Design review of the part built by this model. Coordinates are the model's own, in mm. A direction names the side the tool comes from. Give positions to 0.01 mm unless a question says otherwise; leave off trailing zeros. Order: outer loops, then holes, each group sorted by start corner. A loop starts at its lowest first (then second) coordinate and runs counter-clockwise, first axis right, second up. Notation, with made-up numbers: (-33.5, 82) -> (8.5, 82) arc R30 cw to (8.5, 106) -> close; hole circle Ø10 at (27.5, 12.25). An arc over 180 degrees is marked (long way). One line per item, written item: value.
from build123d import *

# Parameters (mm, degrees)
SKETCH4_W              = 63.5
SKETCH4_H              = 54.9275
BASE_FLANGE1_DEPTH     = 1.905
SKETCHED_START         = -31.75
SKETCHED_BEND3_DEPTH   = 63.5
SKETCHED_BEND3_2_DEPTH = 63.5
CUT_EXTRUDE2_REACH     = 51.835
SKETCH20_R             = 2


# Read off the part's stored shape, not the designer's step: Sketched Bend3
# Sheet-metal steps are written as plain solids
with BuildPart() as part:
    # Sketch4 → Base-Flange1 (new body)
    with BuildSketch(Plane(origin=(0, 0, 0), x_dir=(0, 0, -1), z_dir=(1, 0, 0))):
        Rectangle(SKETCH4_W, SKETCH4_H)
    extrude(amount=-BASE_FLANGE1_DEPTH)

    # Sketched Bend3 outline → Sketched Bend3 (cut)
    with BuildSketch(Plane.XY.offset(SKETCHED_START)):
        with BuildLine():
            ThreePointArc((0, -18.310223013), (-1.375727285, -17.359629491), (-1.905, -15.7734))
            Line((-1.905, -15.7734), (-1.905, -27.46375))
            Line((-1.905, -27.46375), (0, -27.46375))
            Line((0, -27.46375), (0, -18.310223013))
        make_face()
        with BuildLine():
            Line((-1.905, 27.46375), (-1.905, 16.0909))
            ThreePointArc((-1.905, 16.0909), (-1.375727285, 17.677129491), (0, 18.627723013))
            Line((0, 18.627723013), (0, 27.46375))
            Line((0, 27.46375), (-1.905, 27.46375))
        make_face()
    extrude(amount=SKETCHED_BEND3_DEPTH, mode=Mode.SUBTRACT)

    # Sketched Bend3 2 outline → Sketched Bend3 2 (add)
    with BuildSketch(Plane.XY.offset(SKETCHED_START)):
        with BuildLine():
            Line((0, -15.7734), (0, -18.310223013))
            ThreePointArc((0, -18.310223013), (0.364592683, -18.388674577), (0.7366, -18.415))
            Line((0.7366, -18.415), (9.773717924, -18.415))
            Line((9.773717924, -18.415), (9.773717924, -16.51))
            Line((9.773717924, -16.51), (0.7366, -16.51))
            ThreePointArc((0.7366, -16.51), (0.215745145, -16.294254855), (0, -15.7734))
        make_face()
        with BuildLine():
            ThreePointArc((0.7366, 18.7325), (0.364592683, 18.706174577), (0, 18.627723013))
            Line((0, 18.627723013), (0, 16.0909))
            ThreePointArc((0, 16.0909), (0.215745145, 16.611754855), (0.7366, 16.8275))
            Line((0.7366, 16.8275), (9.456217924, 16.8275))
            Line((9.456217924, 16.8275), (9.456217924, 18.7325))
            Line((9.456217924, 18.7325), (0.7366, 18.7325))
        make_face()
    extrude(amount=SKETCHED_BEND3_2_DEPTH)

    # Cut-Extrude2: up to this face of the body (flat: up to its plane)
    cut_extrude2_end = Plane(part.part.faces().sort_by_distance((5.255158962, -18.415, 0))[0])
    # Sketch20 → Cut-Extrude2 (cut, up to the picked face)
    with BuildSketch(Plane(origin=(0, 18.7325, 0), x_dir=(1, 0, 0), z_dir=(0, 1, 0)), mode=Mode.PRIVATE) as cut_extrude2_sk1:
        with Locations(Location((5.08, -6.35, 0), (0, 0, 180))):
            Circle(SKETCH20_R)
    cut_extrude2_tool1 = split(extrude(cut_extrude2_sk1.sketch, amount=-CUT_EXTRUDE2_REACH, mode=Mode.PRIVATE), bisect_by=cut_extrude2_end, keep=Keep.BOTH, mode=Mode.PRIVATE)
    # Sketch20 → Cut-Extrude2 (cut, up to the picked face)
    with BuildSketch(Plane(origin=(0, 18.7325, 0), x_dir=(1, 0, 0), z_dir=(0, 1, 0)), mode=Mode.PRIVATE) as cut_extrude2_sk2:
        with Locations(Location((5.08, 0, 0), (0, 0, 180))):
            Circle(SKETCH20_R)
    cut_extrude2_tool2 = split(extrude(cut_extrude2_sk2.sketch, amount=-CUT_EXTRUDE2_REACH, mode=Mode.PRIVATE), bisect_by=cut_extrude2_end, keep=Keep.BOTH, mode=Mode.PRIVATE)
    # Sketch20 → Cut-Extrude2 (cut, up to the picked face)
    with BuildSketch(Plane(origin=(0, 18.7325, 0), x_dir=(1, 0, 0), z_dir=(0, 1, 0)), mode=Mode.PRIVATE) as cut_extrude2_sk3:
        with Locations(Location((5.08, 6.35, 0), (0, 0, 180))):
            Circle(SKETCH20_R)
    cut_extrude2_tool3 = split(extrude(cut_extrude2_sk3.sketch, amount=-CUT_EXTRUDE2_REACH, mode=Mode.PRIVATE), bisect_by=cut_extrude2_end, keep=Keep.BOTH, mode=Mode.PRIVATE)
    # Sketch20 → Cut-Extrude2 (cut, up to the picked face)
    with BuildSketch(Plane(origin=(0, 18.7325, 0), x_dir=(1, 0, 0), z_dir=(0, 1, 0)), mode=Mode.PRIVATE) as cut_extrude2_sk4:
        with Locations(Location((5.08, 12.7, 0), (0, 0, 180))):
            Circle(SKETCH20_R)
    cut_extrude2_tool4 = split(extrude(cut_extrude2_sk4.sketch, amount=-CUT_EXTRUDE2_REACH, mode=Mode.PRIVATE), bisect_by=cut_extrude2_end, keep=Keep.BOTH, mode=Mode.PRIVATE)
    # Sketch20 → Cut-Extrude2 (cut, up to the picked face)
    with BuildSketch(Plane(origin=(0, 18.7325, 0), x_dir=(1, 0, 0), z_dir=(0, 1, 0)), mode=Mode.PRIVATE) as cut_extrude2_sk5:
        with Locations(Location((5.08, 19.05, 0), (0, 0, 180))):
            Circle(SKETCH20_R)
    cut_extrude2_tool5 = split(extrude(cut_extrude2_sk5.sketch, amount=-CUT_EXTRUDE2_REACH, mode=Mode.PRIVATE), bisect_by=cut_extrude2_end, keep=Keep.BOTH, mode=Mode.PRIVATE)
    # Sketch20 → Cut-Extrude2 (cut, up to the picked face)
    with BuildSketch(Plane(origin=(0, 18.7325, 0), x_dir=(1, 0, 0), z_dir=(0, 1, 0)), mode=Mode.PRIVATE) as cut_extrude2_sk6:
        with Locations(Location((5.08, -12.7, 0), (0, 0, 180))):
            Circle(SKETCH20_R)
    cut_extrude2_tool6 = split(extrude(cut_extrude2_sk6.sketch, amount=-CUT_EXTRUDE2_REACH, mode=Mode.PRIVATE), bisect_by=cut_extrude2_end, keep=Keep.BOTH, mode=Mode.PRIVATE)
    # Sketch20 → Cut-Extrude2 (cut, up to the picked face)
    with BuildSketch(Plane(origin=(0, 18.7325, 0), x_dir=(1, 0, 0), z_dir=(0, 1, 0)), mode=Mode.PRIVATE) as cut_extrude2_sk7:
        with Locations(Location((5.08, -19.05, 0), (0, 0, 180))):
            Circle(SKETCH20_R)
    cut_extrude2_tool7 = split(extrude(cut_extrude2_sk7.sketch, amount=-CUT_EXTRUDE2_REACH, mode=Mode.PRIVATE), bisect_by=cut_extrude2_end, keep=Keep.BOTH, mode=Mode.PRIVATE)
    add(cut_extrude2_tool1.solids().sort_by(Axis((5.08, 18.7325, 6.35), (0, -1, 0)))[0], mode=Mode.SUBTRACT)
    add(cut_extrude2_tool2.solids().sort_by(Axis((5.08, 18.7325, 0), (0, -1, 0)))[0], mode=Mode.SUBTRACT)
    add(cut_extrude2_tool3.solids().sort_by(Axis((5.08, 18.7325, -6.35), (0, -1, 0)))[0], mode=Mode.SUBTRACT)
    add(cut_extrude2_tool4.solids().sort_by(Axis((5.08, 18.7325, -12.7), (0, -1, 0)))[0], mode=Mode.SUBTRACT)
    add(cut_extrude2_tool5.solids().sort_by(Axis((5.08, 18.7325, -19.05), (0, -1, 0)))[0], mode=Mode.SUBTRACT)
    add(cut_extrude2_tool6.solids().sort_by(Axis((5.08, 18.7325, 12.7), (0, -1, 0)))[0], mode=Mode.SUBTRACT)
    add(cut_extrude2_tool7.solids().sort_by(Axis((5.08, 18.7325, 19.05), (0, -1, 0)))[0], mode=Mode.SUBTRACT)


solid = part.part
Item 1: Draft analysis for pull direction Y (two halves, no side actions). For faces 3 (the flat face through (7.3, -16.51, -0.4)), 4 (the flat face through (8, 18.732, 0)), 5 (the flat face through (9.774, -17, 0)), 6 (the flat face through (2, 16.828, 0)), state which applies: pulls with the +Y half, pulls with the -Y half, needs draft (parallel to the pull), parting line crosses it, or undercut.
Returned:
face 3: undercut
face 4: pulls with the +Y half
face 5: needs draft
face 6: undercut
Item 2: Add section A-A on z = 19.05. Give the boundary of the cut face in (x, y) (1 decimal), plus the area to 3 significant figures.
Returned:
outline: (-1.9, -15.8) arc R2.6 ccw to (0.7, -18.4) -> (3.1, -18.4) -> (3.1, -16.5) -> (0.7, -16.5) arc R0.7 cw to (0, -15.8) -> (0, 16.1) arc R0.7 cw to (0.7, 16.8) -> (3.1, 16.8) -> (3.1, 18.7) -> (0.7, 18.7) arc R2.6 ccw to (-1.9, 16.1) -> close; (7.1, -18.4) -> (9.8, -18.4) -> (9.8, -16.5) -> (7.1, -16.5) -> close; (7.1, 16.8) -> (9.5, 16.8) -> (9.5, 18.7) -> (7.1, 18.7) -> close
area: 89.4 mm²
Item 3: Add section C-C on z = -18. Give the boundary of the cut face in (x, y) (1 decimal), plus the area to 3 significant figures.
Returned:
outline: (-1.9, -15.8) arc R2.6 ccw to (0.7, -18.4) -> (3.4, -18.4) -> (3.4, -16.5) -> (0.7, -16.5) arc R0.7 cw to (0, -15.8) -> (0, 16.1) arc R0.7 cw to (0.7, 16.8) -> (3.4, 16.8) -> (3.4, 18.7) -> (0.7, 18.7) arc R2.6 ccw to (-1.9, 16.1) -> close; (6.8, -18.4) -> (9.8, -18.4) -> (9.8, -16.5) -> (6.8, -16.5) -> close; (6.8, 16.8) -> (9.5, 16.8) -> (9.5, 18.7) -> (6.8, 18.7) -> close
area: 91.7 mm²
Item 4: Machinability: for faces 1 (the cylindrical face through (4.005, -17.449, -4.664)), 2 (the flat face through (0, 0, 0)), which of the approach directions +Z, -Z, +X, -X, +Y, -Y give a long, thin tool a straight path to every point of the face, cutting with its end or side? Answer none if there is none.
Returned:
face 1: +Y, -Y
face 2: +Z, -Z, +X
Item 5: To check wall thickness, follow line 1 along Y through (x, z) = (2.5, 8.5) (1 decimal); line 2 along X through (y, z) = (-14.5, 29) (3 decimals); line 3 along X through (y, z) = (17.5, -14.5). State the ranges of each line that lie inside material, in increasing order. Write a range as from..to.
Returned:
line 1: -18.4..-16.5, 16.8..18.7
line 2: -1.905..0
line 3: -1.5..4.21, 5.95..9.46
Item 6: Clearance check with flat-ended pins moving along their axes: P1, Ø1.5, axis at y = 18, z = -9, coming from the +X side; P2, Ø9.5, axis at y = 7.5, z = 8, coming from the +X side. State where each tip first meets the part, or that it passes through.
Returned:
P1: x = 9.46
P2: x = 0
Item 7: Add section D-D on y = -14. Give the boundary of the cut face in (x, z) (3 decimals), plus the area to 3 significant figures.
Returned:
outline: (-1.905, -31.75) -> (0, -31.75) -> (0, 31.75) -> (-1.905, 31.75) -> close
area: 121 mm²
Item 8: Add section B-B on z = -25. Give the boundary of the cut face in (x, y) (1 decimal), plus the area to 3 significant figures.
Returned:
outline: (-1.9, -15.8) arc R2.6 ccw to (0.7, -18.4) -> (9.8, -18.4) -> (9.8, -16.5) -> (0.7, -16.5) arc R0.7 cw to (0, -15.8) -> (0, 16.1) arc R0.7 cw to (0.7, 16.8) -> (9.5, 16.8) -> (9.5, 18.7) -> (0.7, 18.7) arc R2.6 ccw to (-1.9, 16.1) -> close
area: 105 mm²
